For this review, take the finished solid that the model builds, in its own axes (mm). Give positions to 0.01 mm unless a question says otherwise; leave off trailing zeros. Write each loop counter-clockwise with the first axis right and the second up, starting at its lowest first coordinate (ties: lowest second). Pieces come first, ordered by that corner, then holes. Notation, with made-up numbers: (13, 68) -> (46, 68) arc R26 cw to (46, 87) -> close; hole circle Ø2 at (1, 87.25). An arc over 180 degrees is marked (long way). Return JSON: item names as keys, results as strings.
from build123d import *

# Parameters (mm, degrees)
EXTRUDE1_DEPTH     = 4.7625
SKETCH2_R          = 3.125
CUT_EXTRUDE1_DEPTH = 5.7625


with BuildPart() as part:
    # Sketch1 → Extrude1 (new body)
    with BuildSketch(Plane.XY):
        Polygon((-230, 0), (230, 0), (230, 25.4), (12.7, 25.4), (12.7, 450), (-12.7, 450), (-12.7, 25.4), (-230, 25.4), align=None)
    extrude(amount=EXTRUDE1_DEPTH)

    # Sketch2 → Cut-Extrude1 (cut, through all)
    with BuildSketch(Plane.XY.offset(4.7625)):
        with Locations((215, 12.7)):
            Circle(SKETCH2_R)
        with Locations((-215, 12.7)):
            Circle(SKETCH2_R)
        with Locations((0, 435)):
            Circle(SKETCH2_R)
    extrude(amount=-CUT_EXTRUDE1_DEPTH, mode=Mode.SUBTRACT)


solid = part.part
1. For pin 1 (1.4 mm diameter, centred on y = 254, z = 3.5, fed in from -X); pin 2 (2 mm diameter, centred on y = 157.5, z = 4, fed in from +X); pin 3 (1.4 mm diameter, centred on x = -112, z = 3, fed in from +Y), all flat-tipped, find the tip position at first contact; note any pin that passes through.
Results found:
{"pin 1": "stops at x = -12.7", "pin 2": "stops at x = 12.7", "pin 3": "stops at y = 25.4"}
2. Add section A-A, the plane z = 2.6. State the section outline as (x, y) points (3 decimals), plus the area to 3 significant figures.
Results found:
{"outline": "(-230, 0) -> (230, 0) -> (230, 25.4) -> (12.7, 25.4) -> (12.7, 450) -> (-12.7, 450) -> (-12.7, 25.4) -> (-230, 25.4) -> close; hole circle Ø6.25 at (-215, 12.7); hole circle Ø6.25 at (0, 435); hole circle Ø6.25 at (215, 12.7)", "area": "22,400 mm²"}
3. Add section C-C, the plane x = 66. State the section outline as (y, z) points.
Results found:
{"outline": "(0, 0) -> (25.4, 0) -> (25.4, 4.76) -> (0, 4.76) -> close"}
4. Add section B-B, the plane y = 60.5. State the section outline as (x, z) points, plus the area to 3 significant figures.
Results found:
{"outline": "(-12.7, 0) -> (12.7, 0) -> (12.7, 4.76) -> (-12.7, 4.76) -> close", "area": "121 mm²"}
5. To check wall thickness, follow probe 1 along Y at (x, z) = (-215, 1.7) (3 decimals); probe 2 along Y at (x, z) = (0, 1.45) (3 decimals); probe 3 along X at (y, z) = (435, 2.85) (3 decimals). State the ranges of each line that lie inside material, in increasing order.
Results found:
{"probe 1": "y = 0 to 9.575, 15.825 to 25.4", "probe 2": "y = 0 to 431.875, 438.125 to 450", "probe 3": "x = -12.7 to -3.125, 3.125 to 12.7"}
